The listing builds one solid part. Answer for the finished solid, in the listing's coordinates (mm). A direction names the side the tool comes from. Round coordinates to 2 decimals unless told otherwise and drop trailing zeros. Loops run counter-clockwise (first coordinate to the right, second up) from the corner with the lowest first, then second, coordinate; pieces in that order, holes last. Notation, with made-up numbers: (65, 9) - (89, 9) arc R26 ccw to (89, 24) - close; hole circle Ø1 at (2.25, 19). An arc over 180 degrees is marked (long way). One line per item, written item: value.
```python
from build123d import *

# Parameters (mm, degrees)
F1_DEPTH = 279.4
F2_R     = 9.165436
F2_R_2   = 7.9375
F3_DEPTH = 101.6
F4_R     = 9.165436
F4_R_2   = 7.9375
F5_DEPTH = 101.6
F6_R     = 3.175
F7_DEPTH = 25.4
F8_R     = 3.175
F9_DEPTH = 25.4


with BuildPart() as f1:
    # F0 (on Top) → F1 (new body)
    with BuildSketch(Plane.XY):
        Polygon((-4.582718, 7.9375), (-9.165436, 0), (-4.582718, -7.9375), (4.582718, -7.9375), (9.165436, 0), (4.582718, 7.9375), align=None)
    extrude(amount=F1_DEPTH)

    # F2 (on face) → F3 (cut)
    with BuildSketch(Plane.XY.offset(279.4)):
        Circle(F2_R)
        Circle(F2_R_2, mode=Mode.SUBTRACT)
    extrude(amount=-F3_DEPTH, mode=Mode.SUBTRACT)

    # F4 (on face) → F5 (cut)
    with BuildSketch(Plane(origin=(0, 0, 0), x_dir=(1, 0, 0), z_dir=(0, 0, -1))):
        Circle(F4_R)
        Circle(F4_R_2, mode=Mode.SUBTRACT)
    extrude(amount=-F5_DEPTH, mode=Mode.SUBTRACT)

    # F6 (on face) → F7 (cut)
    with BuildSketch(Plane(origin=(0, 0, 0), x_dir=(1, 0, 0), z_dir=(0, 0, -1))):
        Circle(F6_R)
    extrude(amount=-F7_DEPTH, mode=Mode.SUBTRACT)

    # F8 (on face) → F9 (cut)
    with BuildSketch(Plane.XY.offset(279.4)):
        Circle(F8_R)
    extrude(amount=-F9_DEPTH, mode=Mode.SUBTRACT)


solid = f1.part
```
1) A cutting plane is placed at B-B on z = 55. Give the vertices of the cut face in (x, y) (1 decimal).
Final values:
outline: circle Ø15.9 at (0, 0)
2) For faces 1 (the flat face through (-6.91, -3.91, 139.17)), 2 (the flat face through (0, 0, 25.4)), 3 (the cylindrical face through (-1.72, -7.75, 229.31)), determine the directions among +Z, -Z, +X, -X, +Y, -Y from which every point of the face is accessible in a straight line to the end or side of a thin tool.
Final values:
face 1: +Z, -Z, -X, -Y
face 2: -Z
face 3: +Z
3) Each of these flat-tipped pins is pushed along its axis until it touches: pin 1 Ø8 at (y, z) = (-2, 86) entering from -X; pin 2 Ø1.2 at (x, y) = (-5, -7) entering from -Z; pin 3 Ø5.5 at (x, y) = (0, 0) entering from +Z. Where does it stop, or does it pass through?
Final values:
pin 1: x = -7.94
pin 2: z = 101.6
pin 3: z = 254
4) A cutting plane is placed at A-A on z = 105. Give the vertices of the cut face in (x, y).
Final values:
outline: (-9.17, 0) - (-4.58, -7.94) - (4.58, -7.94) - (9.17, 0) - (4.58, 7.94) - (-4.58, 7.94) - close
5) For a pull along X with two mould halves and no side action, classify faces 4 (the flat face through (-6.842, 4.024, 139.167)), 5 (the flat face through (6.91, 3.91, 139.17)), 6 (the cylindrical face through (-0.69, 3.1, 12.52)), 7 (the flat face through (3.4, 0.1, 0)) as released by +X, released by -X, zero draft, split by the parting line, or undercut.
Final values:
face 4: released by -X
face 5: released by +X
face 6: undercut
face 7: zero draft
6) Consider L1, parallel to Y at x = 0, z = 262 (1 decimal); L2, parallel to X at y = 4, z = 109. Determine where each line is inside the solid, lowest interval first.
Final values:
L1: -7.9 to -3.2, 3.2 to 7.9
L2: -6.86 to 6.86
